Verification items for the finished model (mm, model axes). A direction names the side the tool comes from. Round coordinates to 2 decimals unless told otherwise and drop trailing zeros. Write each loop counter-clockwise with the first axis right and the second up, starting at its lowest first coordinate (ties: lowest second). Pieces come first, ordered by that corner, then holes. Notation, with made-up numbers: (81, 23) - (135, 23) arc R14 cw to (135, 29) - close; hole circle Ø1 at (21, 21.5). An arc over 180 degrees is marked (long way). Answer as a JSON object with one key per item and string values. Group by question number.
1) Section check C-C (z = 5). Enter the section's corners in (x, y).
2) Mould release check, pull along Y, two halves, no side actions. Record for faces 1 (the cylindrical face through (-30.99, 31.22, 13.18)), 2 (the flat face through (0, 37, 13)), 3 (the conical face through (31.07, -31.3, 25.81)), 4 (the flat face through (-37, 0, 13)): +Y half, -Y half, draft (parallel to the pull), parting line (faces both ways), or undercut.
3) Set-up check for faces 5 (the cylindrical face through (28.363, 28.192, 0.507)), 6 (the flat face through (35.5, 0, 13)), 7 (the conical face through (32.17, 31.91, 25.88)), 8 (the cylindrical face through (31.22, 30.99, 13.18)): record each of +Z, -Z, +X, -X, +Y, -Y from which the full face is reachable in a straight line by a thin tool's end or side.
4) Section check A-A (y = -15.5). Enter the section's corners in (x, z), then the cut area to 3 significant figures.
5) Thickness scan on line 1 (X direction, y = 0, z = 20.5); line 2 (Y direction, x = 30, z = 11). Record the ranges inside material, lowest first.
6) Go/stop test with flat-tipped pins: pin 1 Ø1 at (y, z) = (26.5, 14.5) entering from +X; pin 2 Ø1.5 at (x, z) = (23, 15) entering from -Y. Record where each tip stops, or that it passes through.
7) Section check D-D (y = 1). Enter the section's corners in (x, z), then the cut area to 3 significant figures.
```python
from build123d import *

# Parameters (mm, degrees)
PAD_DEPTH       = 1
PAD001_DEPTH    = 26
POCKET_DEPTH    = 25
POCKET001_DEPTH = 1.001
PAD002_DEPTH    = 0.5
CHAMFER_SIZE    = 0.3
CHAMFER001_SIZE = 0.3
CHAMFER002_SIZE = 0.3
CHAMFER003_SIZE = 0.3


with BuildPart() as part:
    # Sketch → Pad (new body)
    with BuildSketch(Plane.XY):
        with BuildLine():
            Line((-35.5, 20.5), (-35.5, -20.5))
            ThreePointArc((-35.5, -20.5), (-31.106602, -31.106602), (-20.5, -35.5))
            Line((-20.5, -35.5), (20.5, -35.5))
            ThreePointArc((20.5, -35.5), (31.106602, -31.106602), (35.5, -20.5))
            Line((35.5, -20.5), (35.5, 20.5))
            ThreePointArc((35.5, 20.5), (31.106602, 31.106602), (20.5, 35.5))
            Line((20.5, 35.5), (-20.5, 35.5))
            ThreePointArc((-20.5, 35.5), (-31.106602, 31.106602), (-35.5, 20.5))
        make_face()
    extrude(amount=PAD_DEPTH)

    # Sketch001 → Pad001 (join)
    with BuildSketch(Plane.XY):
        with BuildLine():
            Line((-37, 20.5), (-37, -20.5))
            ThreePointArc((-37, -20.5), (-32.167262, -32.167262), (-20.5, -37))
            Line((-20.5, -37), (20.5, -37))
            ThreePointArc((20.5, -37), (32.167262, -32.167262), (37, -20.5))
            Line((37, -20.5), (37, 20.5))
            ThreePointArc((37, 20.5), (32.167262, 32.167262), (20.5, 37))
            Line((20.5, 37), (-20.5, 37))
            ThreePointArc((-20.5, 37), (-32.167262, 32.167262), (-37, 20.5))
        make_face()
    extrude(amount=PAD001_DEPTH)

    # Sketch002 → Pocket (cut)
    with BuildSketch(Plane.XY.offset(1)):
        with BuildLine():
            Line((-35.5, 20.5), (-35.5, -20.5))
            ThreePointArc((-35.5, -20.5), (-31.106602, -31.106602), (-20.5, -35.5))
            Line((-20.5, -35.5), (20.5, -35.5))
            ThreePointArc((20.5, -35.5), (31.106602, -31.106602), (35.5, -20.5))
            Line((35.5, -20.5), (35.5, 20.5))
            ThreePointArc((35.5, 20.5), (31.106602, 31.106602), (20.5, 35.5))
            Line((20.5, 35.5), (-20.5, 35.5))
            ThreePointArc((-20.5, 35.5), (-31.106602, 31.106602), (-35.5, 20.5))
        make_face()
    extrude(amount=POCKET_DEPTH, mode=Mode.SUBTRACT)

    # Sketch003 (on Face19 of Pocket) → Pocket001 (cut, through all)
    with BuildSketch(Plane.XY.offset(1)):
        with BuildLine():
            Line((-31.5, 20.5), (-31.5, -20.5))
            ThreePointArc((-31.5, -20.5), (-28.278175, -28.278175), (-20.5, -31.5))
            Line((-20.5, -31.5), (20.5, -31.5))
            ThreePointArc((20.5, -31.5), (28.278175, -28.278175), (31.5, -20.5))
            Line((31.5, -20.5), (31.5, 20.5))
            ThreePointArc((31.5, 20.5), (28.278175, 28.278175), (20.5, 31.5))
            Line((20.5, 31.5), (-20.5, 31.5))
            ThreePointArc((-20.5, 31.5), (-28.278175, 28.278175), (-31.5, 20.5))
        make_face()
    extrude(amount=-POCKET001_DEPTH, mode=Mode.SUBTRACT)

    # Sketch004 (on Face19 of Pocket001) → Pad002 (join)
    with BuildSketch(Plane.YZ.offset(-35.5)):
        with BuildLine():
            ThreePointArc((-10, 25.5), (-10.7, 24.8), (-10, 24.1))
            Line((-10, 24.1), (10, 24.1))
            ThreePointArc((10, 24.1), (10.7, 24.8), (10, 25.5))
            Line((-10, 25.5), (10, 25.5))
        make_face()
    pad002 = extrude(amount=PAD002_DEPTH)

    # Mirrored: Pad002 across YZ
    add(pad002.mirror(Plane.YZ))

    # Chamfer
    chamfer_edges = [part.edges().sort_by_distance(p)[0] for p in [
        (-35, 0, 25.5),
    ]]
    chamfer(chamfer_edges, length=CHAMFER_SIZE)

    # Chamfer001
    chamfer001_edges = [part.edges().sort_by_distance(p)[0] for p in [
        (35, 0, 25.5),
    ]]
    chamfer(chamfer001_edges, length=CHAMFER001_SIZE)

    # Chamfer002
    chamfer002_edges = [part.edges().sort_by_distance(p)[0] for p in [
        (0, -35.5, 26),
    ]]
    chamfer(chamfer002_edges, length=CHAMFER002_SIZE)

    # Chamfer003
    chamfer003_edges = [part.edges().sort_by_distance(p)[0] for p in [
        (37, 0, 26),
    ]]
    chamfer(chamfer003_edges, length=CHAMFER003_SIZE)


solid = part.part
```
Returned:
{
 "1": {"outline": "(-37, -20.5) arc R16.5 ccw to (-20.5, -37) - (20.5, -37) arc R16.5 ccw to (37, -20.5) - (37, 20.5) arc R16.5 ccw to (20.5, 37) - (-20.5, 37) arc R16.5 ccw to (-37, 20.5) - close; hole (-35.5, -20.5) arc R15 ccw to (-20.5, -35.5) - (20.5, -35.5) arc R15 ccw to (35.5, -20.5) - (35.5, 20.5) arc R15 ccw to (20.5, 35.5) - (-20.5, 35.5) arc R15 ccw to (-35.5, 20.5) - close"},
 "2": {"face 1": "undercut", "face 2": "+Y half", "face 3": "undercut", "face 4": "draft"},
 "3": {"face 5": "+Z, -Z", "face 6": "none", "face 7": "+Z, +X, +Y", "face 8": "+Z"},
 "4": {"outline": "(-37, 0) - (-31.5, 0) - (-31.5, 1) - (-35.5, 1) - (-35.5, 25.7) - (-35.8, 26) - (-36.7, 26) - (-37, 25.7) - close; (31.5, 0) - (37, 0) - (37, 25.7) - (36.7, 26) - (35.8, 26) - (35.5, 25.7) - (35.5, 1) - (31.5, 1) - close", "area": "85.8 mm2"},
 "5": {"line 1": "-37 to -35.5, 35.5 to 37", "line 2": "-33.99 to -32.11, 32.11 to 33.99"},
 "6": {"pin 1": "x = 36.06", "pin 2": "y = -36.91"},
 "7": {"outline": "(-37, 0) - (-31.5, 0) - (-31.5, 1) - (-35.5, 1) - (-35.5, 24.1) - (-35.3, 24.1) - (-35, 24.4) - (-35, 25.2) - (-35.3, 25.5) - (-35.5, 25.5) - (-35.5, 25.7) - (-35.8, 26) - (-36.7, 26) - (-37, 25.7) - close; (31.5, 0) - (37, 0) - (37, 25.7) - (36.7, 26) - (35.8, 26) - (35.5, 25.7) - (35.5, 25.5) - (35.3, 25.5) - (35, 25.2) - (35, 24.4) - (35.3, 24.1) - (35.5, 24.1) - (35.5, 1) - (31.5, 1) - close", "area": "87.0 mm2"}
}
